Check sheet for the drawn part. Datum: minimum x, y, z corner. Units: mm. A direction names the side the tool comes from. Give positions to 0.01 mm unless a question says otherwise; leave off trailing zeros. Loops run counter-clockwise (first coordinate to the right, second up) from the corner with the lowest first, then second, coordinate; pieces in that order, holes last.
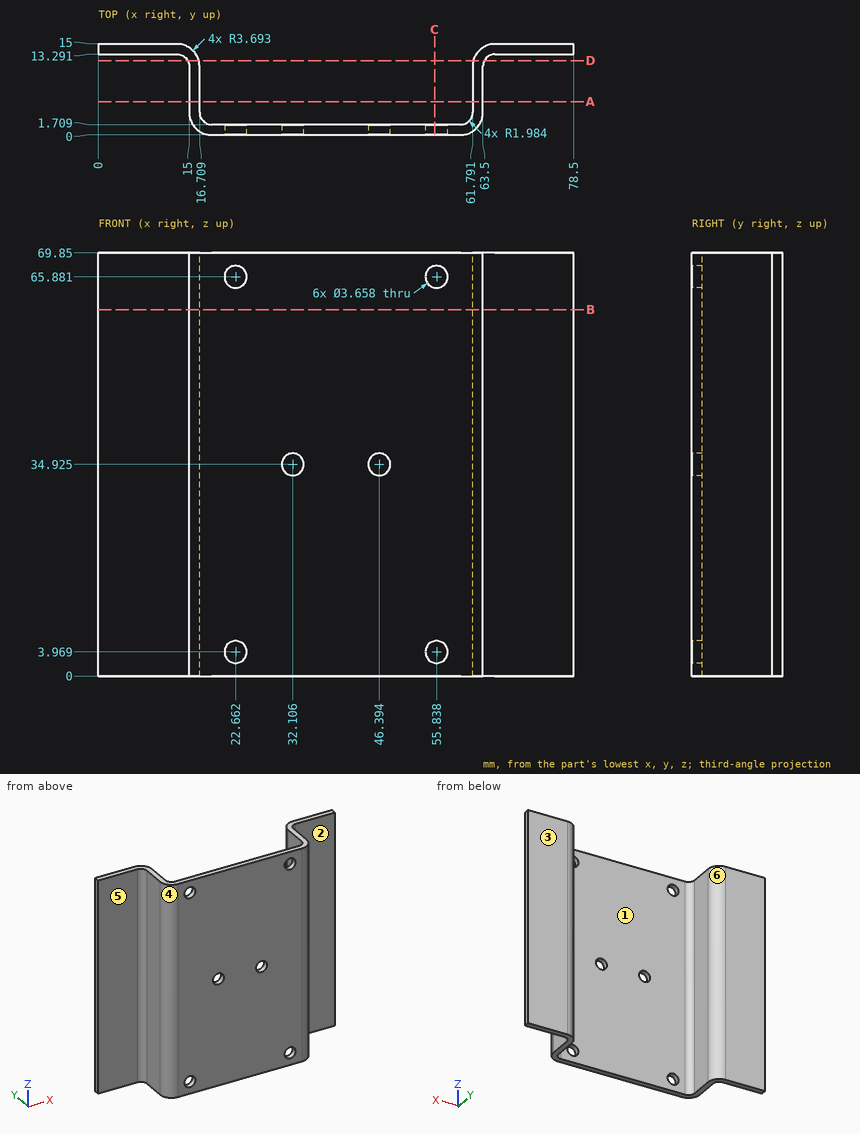
1) Sectioned sample at D-D on y = 12.25. Enter the section's corners in (x, z).
2) Mould release check, pull along X, two halves, no side actions. Record for the marked faces 4, 5 and 6: +X half, -X half, draft (parallel to the pull), parting line (faces both ways), or undercut.
3) Sectioned sample at C-C on x = 55.5. Enter the section's corners in (y, z).
4) Tool access check on the marked faces 1, 2 and 3. Record the directions out of +Z, -Z, +X, -X, +Y, -Y that give a thin tool (end or side, any length) a straight path to the whole face; none if there is none.
5) Scan lines: line 1 along X through (y, z) = (4.75, 40); line 2 along Y through (x, z) = (57, 27); line 3 along Y through (x, z) = (11, 63.5). Record each from-to range of solid material in increasing order.
6) Depth check by flat-ended pin: P1, Ø10.5, axis at x = 6.5, z = 49.5, coming from the -Y side; P2, Ø4, axis at y = 7, z = 16.5, coming from the +X side; P3, Ø3, axis at x = 55.84, z = 65.88, coming from the +Y side; P4, Ø5, axis at x = 45, z = 42, coming from the +Y side. Enter the tip coordinate at first touch or a pass-through.
7) Sectioned sample at B-B on z = 60.5. Enter the section's corners in (x, y), plus the area to 3 significant figures.
8) Sectioned sample at A-A on y = 5.5. Enter the section's corners in (x, z).
Determined:
1. outline: (14.76, 0) - (16.59, 0) - (16.59, 69.85) - (14.76, 69.85) - close; (61.91, 0) - (63.74, 0) - (63.74, 69.85) - (61.91, 69.85) - close
2. face 4: -X half
2. face 5: draft
2. face 6: undercut
3. outline: (0, 0) - (1.71, 0) - (1.71, 2.17) - (0, 2.17) - close; (0, 5.77) - (1.71, 5.77) - (1.71, 64.08) - (0, 64.08) - close; (0, 67.68) - (1.71, 67.68) - (1.71, 69.85) - (0, 69.85) - close
4. face 1: +Z, -Z, +Y
4. face 2: +Z, -Z, +X, -Y
4. face 3: +Z, -Z, +X, -X, +Y
5. line 1: x = 15 to 16.71, 61.79 to 63.5
5. line 2: y = 0 to 1.71
5. line 3: y = 13.29 to 15
6. P1: stops at y = 13.29
6. P2: stops at x = 63.5
6. P3: passes through
6. P4: stops at y = 1.71
7. outline: (0, 13.29) - (13.02, 13.29) arc R1.98 cw to (15, 11.31) - (15, 3.69) arc R3.69 ccw to (18.69, 0) - (59.81, 0) arc R3.69 ccw to (63.5, 3.69) - (63.5, 11.31) arc R1.98 cw to (65.48, 13.29) - (78.5, 13.29) - (78.5, 15) - (65.48, 15) arc R3.69 ccw to (61.79, 11.31) - (61.79, 3.69) arc R1.98 cw to (59.81, 1.71) - (18.69, 1.71) arc R1.98 cw to (16.71, 3.69) - (16.71, 11.31) arc R3.69 ccw to (13.02, 15) - (0, 15) - close
7. area: 171 mm2
8. outline: (15, 0) - (16.71, 0) - (16.71, 69.85) - (15, 69.85) - close; (61.79, 0) - (63.5, 0) - (63.5, 69.85) - (61.79, 69.85) - close
